Design review of the part built by this model. Coordinates are the model's own, in mm. A direction names the side the tool comes from. Coordinates: 2 decimals unless noted, no trailing zeros. Write each loop counter-clockwise with the first axis right and the second up, starting at its lowest first coordinate (ties: lowest second). Pieces come first, ordered by that corner, then holes. Notation, with made-up numbers: (35.5, 62) -> (89.5, 62) arc R24 cw to (89.5, 98) -> close; hole circle Ø4 at (68, 3). An arc over 180 degrees is marked (long way). One line per question, with ' | ' between items. Start each with the question number.
Q1. Add section C-C on x = 0. State the section outline as (y, z) points.
Q2. For P1, Ø1, axis at y = 6.5, z = 4, coming from the -X side; P2, Ø9.5, axis at x = -3, z = -2, coming from the -Y side; P3, Ø12, axis at x = -7, z = -17, coming from the +Y side, all flat-tipped, find the tip position at first contact; note any pin that passes through.
Q3. Add section B-B on y = 7.25. State the section outline as (x, z) points, and give its area (3 significant figures).
Q4. Draft analysis for pull direction Z (two halves, no side actions). For faces 1 (the flat face through (2, 12.5, -6)), 2 (the cylindrical face through (-11.79, -1.23, -0.52)), 3 (the cylindrical face through (-1.172, 4.895, 8.923)), 4 (the flat face through (-11, 4.5, -5)), state which applies: pulls with the +Z half, pulls with the -Z half, needs draft (parallel to the pull), parting line crosses it, or undercut.
Q5. For faces 5 (the cylindrical face through (-16.087, 3.021, -14.405)), 6 (the flat face through (0, 0, 0)), 7 (the cylindrical face through (-11.79, 14.95, 0.52)), list the 3-axis set-ups (+Z, -Z, +X, -X, +Y, -Y) from which the entire face can be reached by the end or side of a thin tool; tool diameter is ignored.
Q6. Wall thickness on probe 1 along Z at (x, y) = (0, 8); probe 2 along Z at (x, y) = (14.6, 3.95); probe 3 along X at (y, z) = (2, -3): over which ranges is each line inside the solid? List them lowest first.
Q7. Add section A-A on z = 14.6. State the section outline as (x, y) points, and give its area (3 significant figures).
Q8. Add section D-D on x = -14.6. State the section outline as (y, z) points, and give its area (3 significant figures).
Autodesk Inventor part; units mm, degrees
ref_plane "YZ Plane" through (0, 0, 0) normal (1, 0, 0) x (0, 1, 0)
ref_plane "XZ Plane" through (0, 0, 0) normal (0, 1, 0) x (-1, 0, 0)
ref_plane "XY Plane" through (0, 0, 0) normal (0, 0, 1) x (1, 0, 0)
sketch "Skizze1" plane through (0, 0, 0) normal (0, 1, 0) x (-1, 0, 0)
  circle A0 centre (0, 0) radius 25.4
  dimension "d0" = 50.8
extrude "Extrusion1" add sketch "Skizze1" along normal blind 4.5
sketch "Skizze2" plane through (0, 0, 0) normal (0, -1, 0) x (1, 0, 0)
  circle A0 centre (0, 0) radius 25.4
  line L0 (-14.6, 14.6) -> (14.6, 14.6) construction
  line L1 (14.6, 14.6) -> (14.6, -14.6) construction
  line L2 (14.6, -14.6) -> (-14.6, -14.6) construction
  line L3 (-14.6, -14.6) -> (-14.6, 14.6) construction
  line L4 (0, 0) -> (14.6, 0) construction
  line L5 (0, 0) -> (0, 14.6) construction
  dimension "d3" = 29.2
  dimension "d4" = 29.2
hole "Bohrung1" at (-14.6, 0, 14.6) at (14.6, 0, 14.6) at (14.6, 0, -14.6) at (-14.6, 0, -14.6) direction (0, 1, 0) diameter 3 end through all countersink diameter 6 countersink angle 90
sketch "Skizze3" plane through (0, 0, 0) normal (0, -1, 0) x (1, 0, 0)
  circle A0 centre (0, 0) radius 25.4
  circle A1 centre (0, 0) radius 11.8
  dimension "d12" = 23.6
extrude "Extrusion2" add sketch "Skizze3" along normal blind 2.5 contours A1
sketch "Skizze4" plane through (0, 4.5, 0) normal (0, 1, 0) x (1, 0, 0)
  circle A0 centre (0, 0) radius 25.4
  circle A1 centre (0, 0) radius 25.4
  circle A2 centre (0, 0) radius 11.8
  dimension "d15" = 23.6
extrude "Extrusion3" add sketch "Skizze4" along normal blind 21.2 contours A2
sketch "Skizze5" plane through (0, -2.5, 0) normal (0, -1, 0) x (1, 0, 0)
  circle A0 centre (0, 0) radius 11.8
  circle A1 centre (0, 0) radius 9
  circle A2 centre (0, 0) radius 6
  dimension "d18" = 18
  dimension "d19" = 12
extrude "Extrusion4" cut sketch "Skizze5" against normal blind 15 contours A1
move faces "Verschieben1" translate (0, 2.5, 0) faces at (-0.7092, -2.5, 1.4219)
properties part number "anschluss_strom"
Output values:
1) outline: (-2.5, -11.8) -> (0, -11.8) -> (0, -25.4) -> (4.5, -25.4) -> (4.5, -11.8) -> (25.7, -11.8) -> (25.7, 11.8) -> (4.5, 11.8) -> (4.5, 25.4) -> (0, 25.4) -> (0, 11.8) -> (-2.5, 11.8) -> (-2.5, 9) -> (12.5, 9) -> (12.5, 6) -> (0, 6) -> (0, -6) -> (12.5, -6) -> (12.5, -9) -> (-2.5, -9) -> close
2) P1: stops at x = -11.27 | P2: stops at y = 0 | P3: stops at y = 4.5
3) outline: circle Ø23.6 at (0, 0); circle Ø12 at (0, 0); hole circle Ø18 at (0, 0) | area: 296 mm2
4) face 1: undercut | face 2: parting line crosses it | face 3: undercut | face 4: needs draft
5) face 5: +Y, -Y | face 6: -Y | face 7: +Y
6) probe 1: z = -11.8 to -9, -6 to 6, 9 to 11.8 | probe 2: z = -20.78 to -16.1, -13.1 to 13.1, 16.1 to 20.78 | probe 3: x = -25.22 to -8.49, -5.2 to 5.2, 8.49 to 25.22
7) outline: (-20.78, 0) -> (-17.6, 0) -> (-16.1, 1.5) -> (-16.1, 4.5) -> (-20.78, 4.5) -> close; (-13.1, 1.5) -> (-11.6, 0) -> (11.6, 0) -> (13.1, 1.5) -> (13.1, 4.5) -> (-13.1, 4.5) -> close; (16.1, 1.5) -> (17.6, 0) -> (20.78, 0) -> (20.78, 4.5) -> (16.1, 4.5) -> close | area: 156 mm2
8) outline: (0, -20.78) -> (4.5, -20.78) -> (4.5, -16.1) -> (1.5, -16.1) -> (0, -17.6) -> close; (0, -11.6) -> (1.5, -13.1) -> (4.5, -13.1) -> (4.5, 13.1) -> (1.5, 13.1) -> (0, 11.6) -> close; (0, 17.6) -> (1.5, 16.1) -> (4.5, 16.1) -> (4.5, 20.78) -> (0, 20.78) -> close | area: 156 mm2
